```python
from build123d import *

# Parameters (mm, degrees)
SKETCH_1_W          = 76.96
SKETCH_1_H          = 39.22
SKETCH_1_R          = 0.9
SKETCH_1_W_2        = 18
SKETCH_1_H_2        = 3
SKETCH_1_W_3        = 18.6
SKETCH_1_H_3        = 17.9
EXTRUDE_1_DEPTH     = 1.6
SKETCH_2_R          = 0.75
CUT_EXTRUDE_1_DEPTH = 1.6
SKETCH_3_W          = 2
SKETCH_3_H          = 3
CUT_EXTRUDE_2_DEPTH = 1.6
SKETCH_5_W          = 8.05
SKETCH_5_H          = 3
CUT_EXTRUDE_3_DEPTH = 10


with BuildPart() as part:
    # 草图1 → 凸台-拉伸1 (new body)
    with BuildSketch(Plane.XY):
        with Locations((0, 1)):
            Rectangle(SKETCH_1_W, SKETCH_1_H)
        with Locations((-16.38, 6.19)):
            Circle(SKETCH_1_R, mode=Mode.SUBTRACT)
        with Locations((16.38, -7.71)):
            Circle(SKETCH_1_R, mode=Mode.SUBTRACT)
        with Locations((5.02, 15.11)):
            Rectangle(SKETCH_1_W_2, SKETCH_1_H_2, mode=Mode.SUBTRACT)
        with Locations((-27.28, -0.76)):
            Rectangle(SKETCH_1_W_3, SKETCH_1_H_3, mode=Mode.SUBTRACT)
        with Locations((27.28, -0.76)):
            Rectangle(SKETCH_1_W_3, SKETCH_1_H_3, mode=Mode.SUBTRACT)
    extrude(amount=EXTRUDE_1_DEPTH)

    # 草图2 → 切除-拉伸1 (cut)
    with BuildSketch(Plane.XY.offset(1.6)):
        with Locations((34.58, 8.79)):
            Circle(SKETCH_2_R)
        with Locations((-34.58, -10.31)):
            Circle(SKETCH_2_R)
    extrude(amount=-CUT_EXTRUDE_1_DEPTH, mode=Mode.SUBTRACT)

    # 草图3 → 切除-拉伸2 (cut)
    with BuildSketch(Plane.XY.offset(1.6)):
        with Locations((6.38, -12.41)):
            Rectangle(SKETCH_3_W, SKETCH_3_H)
        with Locations((-6.38, 10.89)):
            Rectangle(SKETCH_3_W, SKETCH_3_H)
    extrude(amount=-CUT_EXTRUDE_2_DEPTH, mode=Mode.SUBTRACT)

    # 草图5 → 切除-拉伸3 (cut)
    with BuildSketch(Plane.XY.offset(1.6)):
        with Locations((2.915, 4.61)):
            Rectangle(SKETCH_5_W, SKETCH_5_H)
    extrude(amount=-CUT_EXTRUDE_3_DEPTH, mode=Mode.SUBTRACT)


solid = part.part
```
Verification items for the finished model (mm, model axes). A direction names the side the tool comes from. Coordinates: 2 decimals unless noted, no trailing zeros. Loops run counter-clockwise (first coordinate to the right, second up) from the corner with the lowest first, then second, coordinate; pieces in that order, holes last. Notation, with made-up numbers: (55.5, -3.75) - (64.5, -3.75) arc R21 cw to (64.5, 24.25) - close; hole circle Ø1 at (6.25, 66.5). An arc over 180 degrees is marked (long way). Answer as a JSON object with one key per item and string values.
(1) Cross-section at D-D, the plane y = -7.71. Record the boundary of the cut face in (x, z), then the cut area to 3 significant figures.
Response:
{"outline": "(-38.48, 0) - (-36.58, 0) - (-36.58, 1.6) - (-38.48, 1.6) - close; (-17.98, 0) - (15.48, 0) - (15.48, 1.6) - (-17.98, 1.6) - close; (17.28, 0) - (17.98, 0) - (17.98, 1.6) - (17.28, 1.6) - close; (36.58, 0) - (38.48, 0) - (38.48, 1.6) - (36.58, 1.6) - close", "area": "60.7 mm²"}
(2) Scan lines: line 1 along X through (y, z) = (5, 0.9); line 2 along X through (y, z) = (2, 0.15); line 3 along Y through (x, z) = (-3.5, 0.35). Record each from-to range of solid material in increasing order.
Response:
{"line 1": "x = -38.48 to -36.58, -17.98 to -1.11, 6.94 to 17.98, 36.58 to 38.48", "line 2": "x = -38.48 to -36.58, -17.98 to 17.98, 36.58 to 38.48", "line 3": "y = -18.61 to 13.61, 16.61 to 20.61"}
(3) Cross-section at B-B, the plane y = 11. Record the boundary of the cut face in (x, z).
Response:
{"outline": "(-38.48, 0) - (-7.38, 0) - (-7.38, 1.6) - (-38.48, 1.6) - close; (-5.38, 0) - (38.48, 0) - (38.48, 1.6) - (-5.38, 1.6) - close"}
(4) Cross-section at A-A, the plane x = -16.38. Record the boundary of the cut face in (y, z), then the cut area to 3 significant figures.
Response:
{"outline": "(-18.61, 0) - (5.29, 0) - (5.29, 1.6) - (-18.61, 1.6) - close; (7.09, 0) - (20.61, 0) - (20.61, 1.6) - (7.09, 1.6) - close", "area": "59.9 mm²"}
(5) Access from +Z, -Z, +X, -X, +Y, -Y to the whole of each face (thin tool, end or side, straight path). Record for faces 3 (the flat face through (-6, 9.39, 1)), 4 (the flat face through (-1, 1, 0)).
Response:
{"face 3": "+Z, -Z", "face 4": "-Z, +X, -X, +Y, -Y"}
(6) Mould release check, pull along Y, two halves, no side actions. Record for faces 1 (the flat face through (-6, 12.39, 1)), 2 (the flat face through (-1, 1, 1.6)): pulls with the +Y half, pulls with the -Y half, needs draft (parallel to the pull), parting line crosses it, or undercut.
Response:
{"face 1": "undercut", "face 2": "needs draft"}
(7) Cross-section at C-C, the plane z = 0.75. Count the separate pieces of the cut face and the enclosed holes in it, then the cut area to 3 significant figures.
Response:
{"separate pieces": "1", "enclosed holes": "8", "area": "2,250 mm²"}
